Geometry: final body of the model. Coordinates: model frame, mm. A direction names the side the tool comes from. Give positions to 0.01 mm unless a question says otherwise; leave off trailing zeros. Loops run counter-clockwise (first coordinate to the right, second up) from the corner with the lowest first, then second, coordinate; pieces in that order, holes last. Notation, with made-up numbers: (25.25, -14.75) -> (82.25, -14.75) arc R33 cw to (82.25, 17.25) -> close; hole circle Ø11 at (62, 40). An arc over 180 degrees is marked (long way). Answer in a Markdown table with one row per item. Add a question column.
from build123d import *

# Parameters (mm, degrees)
SKETCH1_R           = 1.5
BOSS_EXTRUDE1_DEPTH = 3


with BuildPart() as part:
    # Sketch1 → Boss-Extrude1 (new body)
    with BuildSketch(Plane(origin=(0, 0, 0), x_dir=(1, 0, 0), z_dir=(0, 1, 0))):
        with BuildLine():
            Line((7.951300085, -43.552898009), (7.95129997, -52.052898009))
            Line((7.95129997, -52.052898009), (10.95129997, -52.052898009))
            Line((10.95129997, -52.052898009), (10.95129997, -53.052897806))
            Line((10.95129997, -53.052897806), (7.95129997, -53.052897806))
            Line((7.95129997, -53.052897806), (7.95129997, -58.552897806))
            Line((7.95129997, -58.552897806), (1.95129997, -58.552897806))
            Line((1.95129997, -58.552897806), (1.95129997, -53.052897806))
            Line((1.95129997, -53.052897806), (-1.04870003, -53.052897806))
            Line((-1.04870003, -53.052897806), (-1.04870003, -52.052897806))
            Line((-1.04870003, -52.052897806), (1.95129997, -52.052897806))
            Line((1.95129997, -52.052897806), (1.951300085, -43.552897806))
            Line((1.951300085, -43.552897806), (-2.548699915, -43.552897806))
            ThreePointArc((-2.548699915, -43.552897806), (-5.377127055, -44.724470643), (-6.548699969, -47.552897752))
            Line((-6.548699969, -47.552897752), (-6.548700104, -57.552897752))
            ThreePointArc((-6.548700104, -57.552897752), (-5.377127267, -60.381324893), (-2.548700158, -61.552897806))
            Line((-2.548700158, -61.552897806), (12.451299842, -61.552898009))
            ThreePointArc((12.451299842, -61.552898009), (15.279726982, -60.381325172), (16.451299896, -57.552898064))
            Line((16.451299896, -57.552898064), (16.451300031, -47.552898064))
            ThreePointArc((16.451300031, -47.552898064), (15.279727194, -44.724470923), (12.451300085, -43.552898009))
            Line((12.451300085, -43.552898009), (7.951300085, -43.552898009))
        make_face()
        with Locations((12.451300031, -47.552898009)):
            Circle(SKETCH1_R, mode=Mode.SUBTRACT)
        with Locations((12.451299896, -57.552898009)):
            Circle(SKETCH1_R, mode=Mode.SUBTRACT)
        with Locations((-2.548700104, -57.552897806)):
            Circle(SKETCH1_R, mode=Mode.SUBTRACT)
        with Locations((-2.548699969, -47.552897806)):
            Circle(SKETCH1_R, mode=Mode.SUBTRACT)
    extrude(amount=BOSS_EXTRUDE1_DEPTH)


solid = part.part
(1) Cut plane A-A on x = 8.5. Return the cut outline in (y, z).
(2) Reachability of faces 1 (the flat face through (5, 1, 58.553)), 2 (the flat face through (0, 1, 52.053)), 3 (the flat face through (16.451, 1, 53)) from +Z, -Z, +X, -X, +Y, -Y: full face, straight path, thin tool, end or side. Return the list, or none.
(3) Cut plane C-C on y = 1.95. Return the cut outline in (x, z).
(4) Cut plane D-D on x = -3.5. Return the cut outline in (y, z).
(5) Material intervals for line 1 along X through (y, z) = (0.5, 56); line 2 along X through (y, z) = (1.4, 47.25); line 3 along X through (y, z) = (1.95, 47.75), sorted ascending. Write a range as from..to.
(6) Cut plane B-B on z = 55.25. Return the cut outline in (x, y), then the cut area to 3 significant figures.
Answer list:
| question | item | result |
|---|---|---|
| 1 | outline | (0, 43.55) -> (3, 43.55) -> (3, 52.05) -> (0, 52.05) -> close; (0, 53.05) -> (3, 53.05) -> (3, 61.55) -> (0, 61.55) -> close |
| 2 | face 1 | -Z, +Y, -Y |
| 2 | face 2 | +Y, -Y |
| 2 | face 3 | +Z, -Z, +X, +Y, -Y |
| 3 | outline | (-6.55, 47.55) arc R4 ccw to (-2.55, 43.55) -> (1.95, 43.55) -> (1.95, 52.05) -> (-1.05, 52.05) -> (-1.05, 53.05) -> (1.95, 53.05) -> (1.95, 58.55) -> (7.95, 58.55) -> (7.95, 53.05) -> (10.95, 53.05) -> (10.95, 52.05) -> (7.95, 52.05) -> (7.95, 43.55) -> (12.45, 43.55) arc R4 ccw to (16.45, 47.55) -> (16.45, 57.55) arc R4 ccw to (12.45, 61.55) -> (-2.55, 61.55) arc R4 ccw to (-6.55, 57.55) -> close; hole circle Ø3 at (-2.55, 47.55); hole circle Ø3 at (-2.55, 57.55); hole circle Ø3 at (12.45, 47.55); hole circle Ø3 at (12.45, 57.55) |
| 4 | outline | (0, 43.67) -> (3, 43.67) -> (3, 46.39) -> (0, 46.39) -> close; (0, 48.71) -> (3, 48.71) -> (3, 56.39) -> (0, 56.39) -> close; (0, 58.71) -> (3, 58.71) -> (3, 61.44) -> (0, 61.44) -> close |
| 5 | line 1 | x = -6.55..1.95, 7.95..16.45 |
| 5 | line 2 | x = -6.54..-4.02, -1.08..1.95, 7.95..10.98, 13.92..16.44 |
| 5 | line 3 | x = -6.55..-4.04, -1.06..1.95, 7.95..10.96, 13.94..16.45 |
| 6 | outline | (-6.55, 0) -> (1.95, 0) -> (1.95, 3) -> (-6.55, 3) -> close; (7.95, 0) -> (16.45, 0) -> (16.45, 3) -> (7.95, 3) -> close |
| 6 | area | 51.0 mm² |
